CAD build for the part. Positions are in the model's coordinates, mm. Face numbers are marked on the shaded views. Give positions to 0.01 mm unless a question says otherwise; leave off trailing zeros. Order: outer loops, then holes, each group sorted by start corner. A loop starts at its lowest first (then second) coordinate and runs counter-clockwise, first axis right, second up.
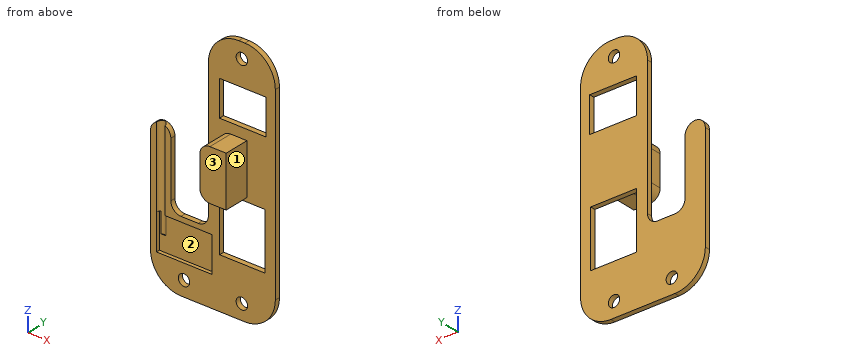
```python
from build123d import *

# Parameters (mm, degrees)
BOSS_EXTRUDE1_DEPTH = 1
SKETCH4_R           = 1.125
CUT_EXTRUDE3_DEPTH  = 6
FILLET1_R           = 6
FILLET2_R           = 2
SKETCH3_R           = 0.85
CUT_EXTRUDE5_DEPTH  = 20
SKETCH6_W           = 11
SKETCH6_H           = 7
CUT_EXTRUDE6_DEPTH  = 0.7
SKETCH7_W           = 9.2
SKETCH7_H           = 7
SKETCH7_W_2         = 9
SKETCH7_H_2         = 11.2
CUT_EXTRUDE7_DEPTH  = 30.733515978
SKETCH8_W           = 5.2
SKETCH8_H           = 10
BOSS_EXTRUDE2_DEPTH = 5
FILLET4_R           = 2


with BuildPart() as part:
    # Sketch1 → Boss-Extrude1 (new body)
    with BuildSketch(Plane(origin=(0, 0, 0), x_dir=(1, 0, 0), z_dir=(0, 1, 0))):
        Polygon((-16.635707691, 24.623874564), (7.964292309, 24.623874564), (7.964292309, -24.376125436), (-5.235707691, -24.376125436), (-5.235707691, 10.623874564), (-12.635707691, 10.623874564), (-12.635707691, -4.376125436), (-16.635707691, -4.376125436), align=None)
    extrude(amount=BOSS_EXTRUDE1_DEPTH)

    # Sketch4 → Cut-Extrude3 (cut)
    with BuildSketch(Plane(origin=(0, 1, 0), x_dir=(1, 0, 0), z_dir=(0, 1, 0))):
        with Locations(Location((-10.035707691, 21.623874564, 0), (0, 0, 270))):
            Circle(SKETCH4_R)
        with Locations(Location((1.364292309, 21.623874564, 0), (0, 0, 270))):
            Circle(SKETCH4_R)
        with Locations(Location((1.364292309, -21.376125436, 0), (0, 0, 270))):
            Circle(SKETCH4_R)
    extrude(amount=-CUT_EXTRUDE3_DEPTH, mode=Mode.SUBTRACT)

    # Fillet1
    fillet1_edges = [part.edges().sort_by_distance(p)[0] for p in [
        (-16.635707691, 0.5, -24.623874564),
        (7.964292309, 0.5, -24.623874564),
        (7.964292309, 0.5, 24.376125436),
        (-5.235707691, 0.5, 24.376125436),
    ]]
    fillet(fillet1_edges, radius=FILLET1_R)

    # Fillet2
    fillet2_edges = [part.edges().sort_by_distance(p)[0] for p in [
        (-5.235707691, 0.5, -10.623874564),
        (-12.635707691, 0.5, -10.623874564),
    ]]
    fillet(fillet2_edges, radius=FILLET2_R)
    fillet2_2_edges = [part.edges().sort_by_distance(p)[0] for p in [
        (-12.635707691, 0.5, 4.376125436),
        (-16.635707691, 0.5, 4.376125436),
    ]]
    fillet(fillet2_2_edges, radius=FILLET2_R - 0.0001)  # a hair under: the kernel refuses the full size

    # Sketch3 → Cut-Extrude5 (cut)
    with BuildSketch(Plane.XY.offset(4.376125436)):
        with Locations((-14.635707691, 0)):
            Circle(SKETCH3_R)
    extrude(amount=-CUT_EXTRUDE5_DEPTH, mode=Mode.SUBTRACT)

    # Sketch6 → Cut-Extrude6 (cut)
    with BuildSketch(Plane.XZ):
        with Locations((-9.985707691, -15.123874564)):
            Rectangle(SKETCH6_W, SKETCH6_H)
    extrude(amount=-CUT_EXTRUDE6_DEPTH, mode=Mode.SUBTRACT)

    # Sketch7 → Cut-Extrude7 (cut, through all)
    with BuildSketch(Plane(origin=(0, 1, 0), x_dir=(1, 0, 0), z_dir=(0, 1, 0))):
        with Locations((1.564292309, -12.876125436)):
            Rectangle(SKETCH7_W, SKETCH7_H)
        with Locations((1.464292309, 9.023874564)):
            Rectangle(SKETCH7_W_2, SKETCH7_H_2)
    extrude(amount=-CUT_EXTRUDE7_DEPTH, mode=Mode.SUBTRACT)

    # Sketch8 → Boss-Extrude2 (add)
    with BuildSketch(Plane.XZ):
        with Locations((-0.235707691, 2.376125436)):
            Rectangle(SKETCH8_W, SKETCH8_H)
    extrude(amount=BOSS_EXTRUDE2_DEPTH)

    # Fillet4
    fillet4_edges = [part.edges().sort_by_distance(p)[0] for p in [
        (-2.835707691, -2.5, 7.376125436),
        (-2.835707691, -2.5, -2.623874564),
    ]]
    fillet(fillet4_edges, radius=FILLET4_R)


solid = part.part
```
Item 1: Drop flat-ended pins along their axis: pin 1 Ø0.8 at (x, y) = (-11.5, 0.5) entering from -Z; pin 2 Ø0.5 at (x, y) = (3.5, 0.5) entering from +Z; pin 3 Ø0.8 at (y, z) = (0.5, 8) entering from -X. Give the stop position or say it passes through.
Item 2: Slice it at B-B (y = -3). Give the cut face in (x, z).
Item 3: Slice it at C-C (z = 19). Give the cut face in (x, y), and give its area (3 significant figures).
Item 4: Two-plate mould, pull along X, no slides. Class the marked faces 1, 2 and 3: released by +X, released by -X, zero draft, split by the parting line, or undercut.
Item 5: Wall check: L1, parallel to X at y = 0.5, z = 9.5; L2, parallel to Y at x = 6, z = -10; L3, parallel to Y at x = -10, z = -17.5. Give the ranges that are in metal, low to high.
Item 6: Slice it at A-A (z = -4). Give the cut face in (x, y).
A:
1. pin 1: stops at z = -24.61
1. pin 2: stops at z = 24.24
1. pin 3: stops at x = -5.24
2. outline: (-2.84, -0.62) arc R2 ccw to (-0.84, -2.62) - (2.36, -2.62) - (2.36, 7.38) - (-0.84, 7.38) arc R2 ccw to (-2.84, 5.38) - close
3. outline: (-5.2, 0) - (7.93, 0) - (7.93, 1) - (-5.2, 1) - close
3. area: 13.1 mm2
4. face 1: released by +X
4. face 2: undercut
4. face 3: zero draft
5. L1: x = -5.24 to -3.04, 6.16 to 7.96
5. L2: y = 0 to 1
5. L3: y = 0.7 to 1
6. outline: (-16.64, 0) - (-15.49, 0) arc R0.85 cw to (-13.79, 0) - (-12.64, 0) - (-12.64, 1) - (-16.64, 1) - close; (-5.24, 0) - (-3.04, 0) - (-3.04, 1) - (-5.24, 1) - close; (5.96, 0) - (7.96, 0) - (7.96, 1) - (5.96, 1) - close
